The listing builds one solid part. Answer for the finished solid, in the listing's coordinates (mm). A direction names the side the tool comes from. Round coordinates to 2 decimals unless told otherwise and drop trailing zeros. Loops run counter-clockwise (first coordinate to the right, second up) from the corner with the lowest first, then second, coordinate; pieces in that order, holes last. Notation, with made-up numbers: (81, 67) - (102, 67) arc R17 ccw to (102, 89) - close; hole circle Ø2 at (14, 82.25). An arc over 180 degrees is marked (long way). One line per item, written item: value.
```python
from build123d import *

# Parameters (mm, degrees)
F1_DEPTH = 100
F2_R     = 5


with BuildPart() as f1:
    # F0 (on Top) → F1 (new body)
    with BuildSketch(Plane.XY):
        Polygon((-49.999979, 349.065976), (-50.000021, -349.066024), (0, -299.066), (49.999979, -349.065976), (50.000021, 349.066024), (0, 299.066), align=None)
    extrude(amount=F1_DEPTH)

    # F2
    f2_edges = [f1.edges().sort_by_distance(p)[0] for p in [
        (50, 2.4e-05, 100),
        (50, 2.4e-05, 0),
        (-50, -2.4e-05, 100),
        (-50, -2.4e-05, 0),
    ]]
    fillet(f2_edges, radius=F2_R)


solid = f1.part
```
1) For a pull along X with two mould halves and no side action, classify faces 4 (the flat face through (24.65, -323.716, 49.3)), 5 (the flat face through (-50, 5, 49)), 6 (the flat face through (-1, 5, 0)) as released by +X, released by -X, zero draft, split by the parting line, or undercut.
Final values:
face 4: undercut
face 5: released by -X
face 6: zero draft
2) Consider L1, parallel to Z at x = 46, y = -294; L2, parallel to X at y = -167, z = 96; L3, parallel to X at y = -310.5, z = 22.5. Determine where each line is inside the solid, lowest interval first.
Final values:
L1: 0.1 to 99.9
L2: -49.9 to 49.9
L3: -50 to -11.43, 11.43 to 50
3) A cutting plane is placed at B-B on x = -9.5. Give the vertices of the cut face in (y, z).
Final values:
outline: (-308.57, 0) - (308.57, 0) - (308.57, 100) - (-308.57, 100) - close
4) For faces 1 (the flat face through (-1, 5, 100)), 2 (the flat face through (25.35, 324.416, 49.3)), 3 (the flat face through (-25.35, -324.416, 49.3)), determine the directions among +Z, -Z, +X, -X, +Y, -Y from which every point of the face is accessible in a straight line to the end or side of a thin tool.
Final values:
face 1: +Z, +X, -X, +Y, -Y
face 2: +Z, -Z, +Y
face 3: +Z, -Z, -Y
5) A cutting plane is placed at C-C on x = 29. Give the vertices of the cut face in (y, z).
Final values:
outline: (-328.07, 0) - (328.07, 0) - (328.07, 100) - (-328.07, 100) - close
6) Each of these flat-tipped pins is pushed along its axis until it touches: pin 1 Ø8 at (x, z) = (11.5, 40) entering from +Y; pin 2 Ø8 at (x, z) = (12.5, 61.5) entering from +Y; pin 3 Ø12 at (x, z) = (34, 10.5) entering from +Y. Where does it stop, or does it pass through?
Final values:
pin 1: y = 314.57
pin 2: y = 315.57
pin 3: y = 339.07
7) A cutting plane is placed at A-A on z = 41. Give the vertices of the cut face in (x, y).
Final values:
outline: (-50, -349.07) - (0, -299.07) - (50, -349.07) - (50, 349.07) - (0, 299.07) - (-50, 349.07) - close
